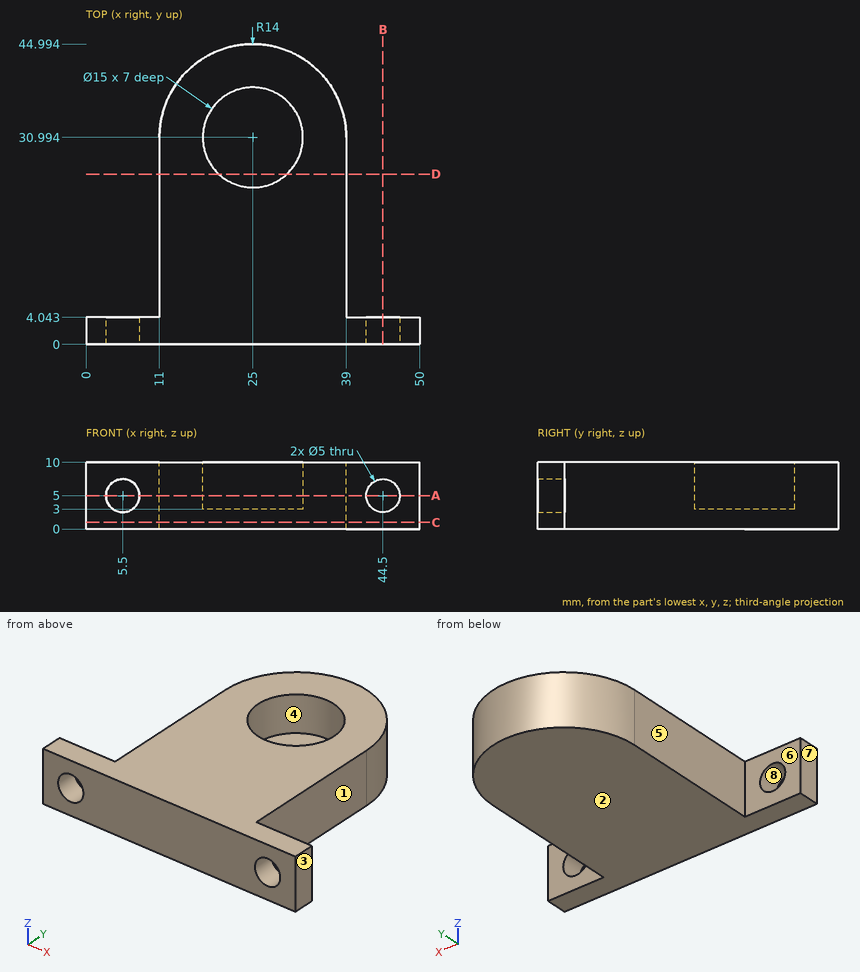
Could you check a few things on this drawing? It's one solid part, dimensions in mm from its lowest x, y, z. A direction names the side the tool comes from. Coordinates: 2 decimals unless noted, no trailing zeros. Order: outer loops, then holes, each group sorted by start corner. A loop starts at its lowest first (then second) coordinate and runs counter-clockwise, first axis right, second up.
1) Imagine slicing it at C-C on z = 1. List the corners of the cut face in (x, y) for me.
2) Will these pins go through, and if not, where does the flat tip stop? pin 1 (5 mm diameter, centred on y = 7.5, z = 2, fed in from +X); pin 2 (4 mm diameter, centred on y = 9.5, z = 2, fed in from -X); pin 3 (3 mm diameter, centred on x = 47, z = 4.5, fed in from +Y); pin 4 (4 mm diameter, centred on x = 44.5, z = 5, fed in from -Y).
3) Imagine slicing it at D-D on y = 25.5. List the corners of the cut face in (x, z) for me (1 decimal).
4) We'd pull the mould along X, two halves only. Please class the marked faces 6, 7 and 8: +X half, -X half, draft (parallel to the pull), parting line (faces both ways), or undercut.
5) Imagine slicing it at B-B on x = 44.5. List the corners of the cut face in (y, z) for me.
6) Imagine slicing it at A-A on z = 5. List the corners of the cut face in (x, y) for me.
7) Which directions (+Z, -Z, +X, -X, +Y, -Y) give clear straight access to the entire face, cutting with the end or side of a thin tool? Please do the marked faces 1, 2, 3, 4 and 5.
8) I need wall thicknesses on line 1 (X direction, y = 1.55, z = 5); line 2 (Y direction, x = 25, z = 7.75); line 3 (Z direction, x = 44.5, y = 2.5). Which ranges of each line are inside material? Lowest first, please.
Response values:
1. outline: (0, 0) - (50, 0) - (50, 4.04) - (39, 4.04) - (39, 30.99) arc R14 ccw to (11, 30.99) - (11, 4.04) - (0, 4.04) - close
2. pin 1: stops at x = 39
2. pin 2: stops at x = 11
2. pin 3: stops at y = 4.04
2. pin 4: passes through
3. outline: (11, 0) - (39, 0) - (39, 10) - (30.1, 10) - (30.1, 3) - (19.9, 3) - (19.9, 10) - (11, 10) - close
4. face 6: draft
4. face 7: -X half
4. face 8: undercut
5. outline: (0, 0) - (4.04, 0) - (4.04, 2.5) - (0, 2.5) - close; (0, 7.5) - (4.04, 7.5) - (4.04, 10) - (0, 10) - close
6. outline: (0, 0) - (3, 0) - (3, 4.04) - (0, 4.04) - close; (8, 0) - (42, 0) - (42, 4.04) - (39, 4.04) - (39, 30.99) arc R14 ccw to (11, 30.99) - (11, 4.04) - (8, 4.04) - close; (47, 0) - (50, 0) - (50, 4.04) - (47, 4.04) - close; hole circle Ø15 at (25, 30.99)
7. face 1: +Z, -Z, +X, +Y
7. face 2: -Z, +X, -X, +Y, -Y
7. face 3: +Z, -Z, +X, +Y, -Y
7. face 4: +Z
7. face 5: +Z, -Z, -X, +Y
8. line 1: x = 0 to 3, 8 to 42, 47 to 50
8. line 2: y = 0 to 23.49, 38.49 to 44.99
8. line 3: z = 0 to 2.5, 7.5 to 10
